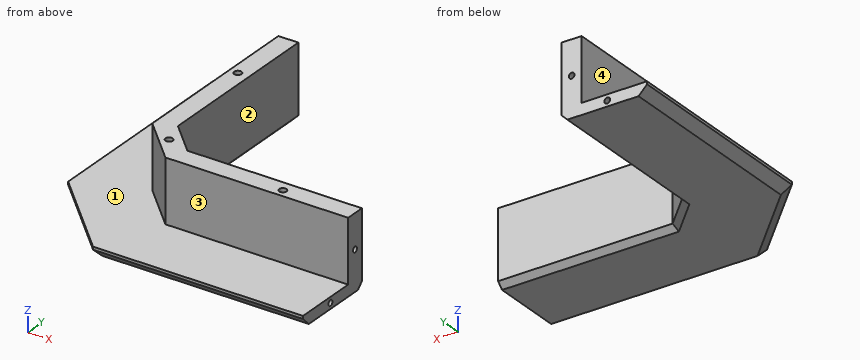
from build123d import *

# Parameters (mm, degrees)
PAD_DEPTH       = 4
PAD001_DEPTH    = 22
CHAMFER_SIZE    = 3
CHAMFER001_SIZE = 2
SKETCH002_R     = 1.3
POCKET_DEPTH    = 15
SKETCH003_R     = 1
POCKET001_DEPTH = 15
SKETCH004_R     = 1
POCKET002_DEPTH = 15


with BuildPart() as part:
    # Sketch → Pad (new body)
    with BuildSketch(Plane.XY):
        Polygon((0, 0), (-73.715729, 0), (-102, 28.284271), (-102, 102), (-72, 102), (-72, 40.710678), (-61.289322, 30), (0, 30), align=None)
    extrude(amount=PAD_DEPTH)

    # Sketch001 (on Face10 of Pad) → Pad001 (join)
    with BuildSketch(Plane.XY.offset(4)):
        Polygon((0, 30), (-61.289322, 30), (-72, 40.710678), (-72, 102), (-79, 102), (-79, 37.811183), (-64.188817, 23), (0, 23), align=None)
    extrude(amount=PAD001_DEPTH)

    # Chamfer
    chamfer_edges = [part.edges().sort_by_distance(p)[0] for p in [
        (-102, 65.142136, 0),
        (-87.857864, 14.142136, 0),
        (-36.857864, 0, 0),
    ]]
    chamfer(chamfer_edges, length=CHAMFER_SIZE)

    # Chamfer001
    chamfer001_edges = [part.edges().sort_by_distance(p)[0] for p in [
        (-72, 71.355339, 0),
        (-66.644661, 35.355339, 0),
        (-30.644661, 30, 0),
    ]]
    chamfer(chamfer001_edges, length=CHAMFER001_SIZE)

    # Sketch002 (on Face18 of Chamfer001) → Pocket (cut)
    with BuildSketch(Plane.XY.offset(26)):
        with Locations((-76, 77)):
            Circle(SKETCH002_R)
        with Locations((-69.473088, 32.526912)):
            Circle(SKETCH002_R)
        with Locations((-25, 26)):
            Circle(SKETCH002_R)
    extrude(amount=-POCKET_DEPTH, mode=Mode.SUBTRACT)

    # Sketch003 (on Face7 of Pocket) → Pocket001 (cut)
    with BuildSketch(Plane.YZ):
        with Locations((26.5, 14)):
            Circle(SKETCH003_R)
        with Locations((14, 2)):
            Circle(SKETCH003_R)
    extrude(amount=-POCKET001_DEPTH, mode=Mode.SUBTRACT)

    # Sketch004 (on Face26 of Pocket001) → Pocket002 (cut)
    with BuildSketch(Plane(origin=(0, 102, 0), x_dir=(-1, 0, 0), z_dir=(0, 1, 0))):
        with Locations((75.5, 14)):
            Circle(SKETCH004_R)
        with Locations((88, 2)):
            Circle(SKETCH004_R)
    extrude(amount=-POCKET002_DEPTH, mode=Mode.SUBTRACT)


solid = part.part
The model under review builds one solid part; all positions refer to its coordinate system, in mm. Face numbers are marked on the shaded views. A direction names the side the tool comes from. Round coordinates to 2 decimals unless told otherwise and drop trailing zeros. Loops run counter-clockwise (first coordinate to the right, second up) from the corner with the lowest first, then second, coordinate; pieces in that order, holes last. Notation, with made-up numbers: M -32.5,69.25 L -5.5,69.25 A29 cw -5.5,103.25 Z; hole C 57.5,-24 d3. An arc over 180 degrees is marked long. Answer as CSV lines item,"result". Start each with the question number.
Item 1: Consider section D-D (y = 77). Write out the cut boundary in (x, z), then the cut area to 4 significant figures.
Item 2: Consider section C-C (x = -80.5). Write out the cut boundary in (y, z).
Item 3: Consider section B-B (y = 52). Write out the cut boundary in (x, z).
Item 4: For the marked faces 1, 2, 3 and 4, list the 3-axis set-ups (+Z, -Z, +X, -X, +Y, -Y) from which the entire face can be reached by the end or side of a thin tool; tool diameter is ignored.
Item 5: Insertion check: P1, Ø2, axis at y = 14, z = 2.5, coming from the +X side; P2, Ø6, axis at x = -19.5, z = 6, coming from the +Y side; P3, Ø10, axis at x = -74, z = 9.5, coming from the -Y side; P4, Ø8, axis at x = -17.5, z = 18.5, coming from the -Y side. Each pin has a flat end and moves straight along its axis. Give the tip position at first contact, or say it passes through.
Item 6: Consider section A-A (z = 6). Write out the cut boundary in (x, y).
Item 7: Wall thickness on line 1 (X direction, y = 59.5, z = 13.75); line 2 (Y direction, x = -25, z = 16); line 3 (Y direction, x = -23.5, z = 11.75): over which ranges is each line inside the solid? List them lowest first. Write a range as [from, to].
Answer:
1,outline,"M -102,3 L -99,0 L -74,0 L -72,2 L -72,26 L -74.7,26 L -74.7,11 L -77.3,11 L -77.3,26 L -79,26 L -79,4 L -102,4 Z"
1,area,"228.5 mm^2"
2,outline,"M 6.78,3 L 11.03,0 L 102,0 L 102,4 L 6.78,4 Z"
3,outline,"M -102,3 L -99,0 L -74,0 L -72,2 L -72,26 L -79,26 L -79,4 L -102,4 Z"
4,face 1,"+Z, -X, -Y"
4,face 2,"+Z, -Z, +X, +Y"
4,face 3,"+Z, +X, -X, -Y"
4,face 4,"+Z, -X, +Y, -Y"
5,P1,"stops at x = 0"
5,P2,"stops at y = 30"
5,P3,"stops at y = 27.81"
5,P4,"stops at y = 23"
6,outline,"M -79,37.81 L -64.19,23 L 0,23 L 0,30 L -61.29,30 L -72,40.71 L -72,102 L -79,102 Z"
7,line 1,"x = [-79, -72]"
7,line 2,"y = [23, 24.7], [27.3, 30]"
7,line 3,"y = [23, 30]"
